Here's how the part is built. I have some questions about the finished solid (model axes, mm). Face numbers are marked on the shaded views. A direction names the side the tool comes from. Round coordinates to 2 decimals unless told otherwise and drop trailing zeros. Loops run counter-clockwise (first coordinate to the right, second up) from the corner with the lowest first, then second, coordinate; pieces in that order, holes last. Notation, with made-up numbers: M 66.25,-33.5 L 96.25,-33.5 A28 ccw 96.25,-9.5 Z; hole C 19.5,42.25 d10. An arc over 180 degrees is marked long. Use a Markdown table: item, result.
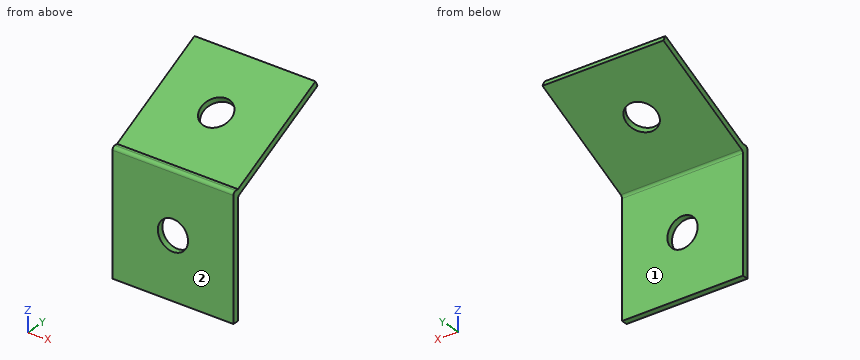
Autodesk Inventor part; units mm, degrees
ref_plane "Work Plane1" through (10, 1, 10) normal (0, 0.4570979, -0.8894164) x (0, 0.8894164, 0.4570979)
ref_plane "YZ Plane" through (0, 0, 0) normal (1, 0, 0) x (0, 1, 0)
ref_plane "XZ Plane" through (0, 0, 0) normal (0, 1, 0) x (-1, 0, 0)
sketch "Sketch1" plane through (0, 0, 0) normal (0, 1, 0) x (-1, 0, 0)
  line L0 (-10, -10) -> (10, -10)
  line L1 (10, -10) -> (10, 10)
  line L2 (10, 10) -> (-10, 10)
  line L3 (-10, 10) -> (-10, -10)
  line L4 (-10, -10) -> (10, 10) construction
  line L5 (10, -10) -> (-10, 10) construction
  point P0 (0, 0)
  dimension "d0" = 20
  dimension "d1" = 20
extrude "Extrusion1" add sketch "Sketch1" along normal blind 1
sketch "Sketch3" plane through (10, 0, 10) normal (1, 0, 0) x (0, 0, -1)
  line L0 (20, 1) -> (0, 1)
  line L1 (0, 1) -> (-0.9142, 2.7788)
  line L2 (0, 1) -> (2, 1) construction
  point P0 (10, 0)
  dimension "d5" = 2
  dimension "d6" = 117.2
ref_plane "Work Plane1" through (10, 1, 10) normal (0, 0.4570979, -0.8894164) x (0, 0.8894164, 0.4570979)
sketch "Sketch4" plane through (10, 1, 10) normal (0, 0.4570979, -0.8894164) x (0, 0.8894164, 0.4570979)
  line L0 (-9.142, -20) -> (0, -20)
  line L1 (0, -20) -> (19, -20)
  line L2 (19, -20) -> (19, 0)
  line L3 (19, 0) -> (0, 0)
  line L4 (0, 0) -> (0, -20)
  point P0 (-5.4604, -10)
  dimension "d7" = 19
  dimension "d8" = 20
extrude "Extrusion2" add sketch "Sketch4" along normal blind 1
sketch "Sketch5" plane through (10, 1, 10) normal (1, 0, 0) x (0, 0.4570979, -0.8894164)
  line L0 (0, 0) -> (1, 0)
  line L1 (1, 0) -> (1, -0.5139)
  line L2 (17.7883, -9.142) -> (0, 0)
  line L3 (1, 0) -> (0, 0)
  line L4 (0, 0) -> (1, -0.5139)
  point P0 (8.4371, -5.4604)
extrude "Extrusion3" add sketch "Sketch5" against normal blind 20
fillet "Fillet1" radius 0.5 2 edges at (0, 1, 8.8757) (0, 0, 10)
sketch "Sketch6" plane through (0, 1, 0) normal (0, 1, 0) x (1, 0, 0)
  circle A0 centre (0, 0) radius 2.5
  dimension "d14" = 5
sketch "Sketch7" plane through (10, 1.4571, 9.1106) normal (0, 0.4570979, -0.8894164) x (-1, 0, 0)
  circle A0 centre (10, 9.5) radius 2.5
  point P0 (10, -5.4604)
  dimension "d15" = 5
extrude "Extrusion4" cut sketch "Sketch6" against normal blind 10
extrude "Extrusion5" cut sketch "Sketch7" against normal blind 10
properties part number "trail 17"
Q1. For the marked faces 1 and 2, which set-ups out of +Z, -Z, +X, -X, +Y, -Y let a thin tool reach every point of the face, with its end or its side?
Return value:
| item | result |
|---|---|
| face 1 | -Z, +X, -X, +Y |
| face 2 | +Z, -Z, +X, -X, -Y |
Q2. Imagine slicing it at D-D, the plane z = -7.25. Please give me the cut outline in (x, y).
Return value:
| item | result |
|---|---|
| outline | M -10,0 L 10,0 L 10,1 L -10,1 Z |
Q3. Imagine slicing it at B-B, the plane x = 4.25. Please give me the cut outline in (y, z).
Return value:
| item | result |
|---|---|
| outline | M 0,-10 L 1,-10 L 1,8.57 A0.5 cw 1.27,9.02 L 18.36,17.8 L 17.9,18.68 L 1,10 L 0.5,10 A0.5 ccw 0,9.5 Z |
Q4. Will these pins go through, and if not, where does the flat tip stop? P1, Ø6, axis at x = 1, y = 9.5, coming from the -Z side; P2, Ø4, axis at x = 0, z = 0, coming from the +Y side; P3, Ø1, axis at x = 3, z = 15, coming from the -Y side; P4, Ø5.5, axis at x = -4.5, z = -3.5, coming from the +Y side.
Return value:
| item | result |
|---|---|
| P1 | stops at z = 11.7 |
| P2 | passes through |
| P3 | stops at y = 9.76 |
| P4 | stops at y = 1 |
Q5. Imagine slicing it at C-C, the plane x = 0. Please give me the cut outline in (y, z), then the cut area to 3 significant figures.
Return value:
| item | result |
|---|---|
| outline | M 0,-10 L 1,-10 L 1,-2.5 L 0,-2.5 Z; M 0,2.5 L 1,2.5 L 1,8.57 A0.5 cw 1.27,9.02 L 7.68,12.31 L 7.23,13.2 L 1,10 L 0.5,10 A0.5 ccw 0,9.5 Z; M 11.67,15.49 L 12.13,14.6 L 18.36,17.8 L 17.9,18.68 Z |
| area | 29.2 mm^2 |
Q6. Imagine slicing it at A-A, the plane z = 0. Please give me the cut outline in (x, y).
Return value:
| item | result |
|---|---|
| outline | M -10,0 L -2.5,0 L -2.5,1 L -10,1 Z; M 2.5,0 L 10,0 L 10,1 L 2.5,1 Z |
Q7. I need wall thicknesses on line 1 (X direction, y = 0.45, z = 0); line 2 (Y direction, x = -3.5, z = 8.25). Which ranges of each line are inside material? Lowest first, please. Write a range as from..to.
Return value:
| item | result |
|---|---|
| line 1 | x = -10..-2.5, 2.5..10 |
| line 2 | y = 0..1 |
